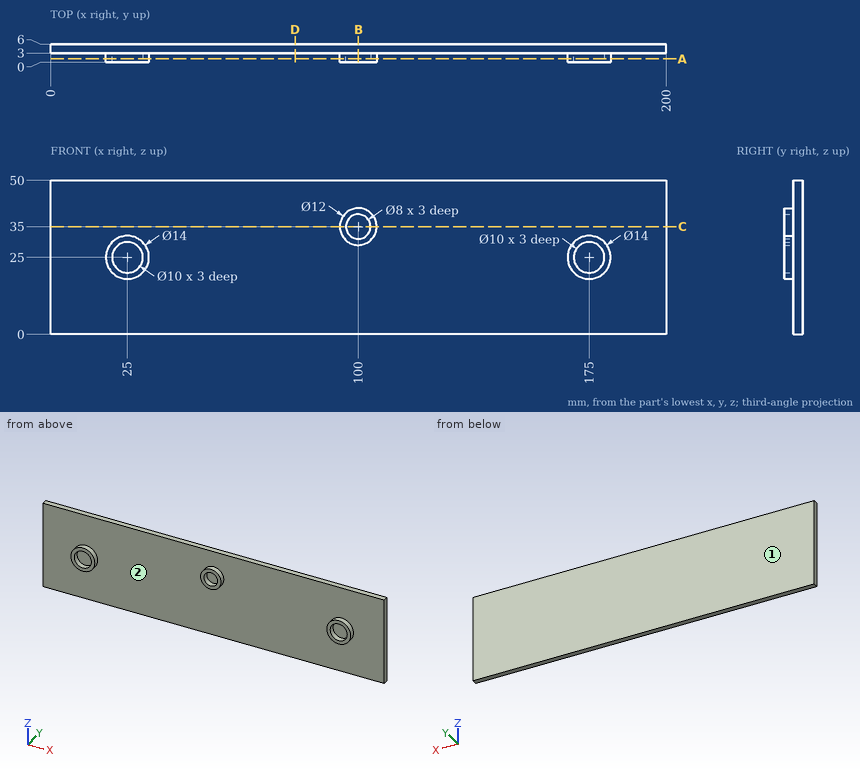
Could you check a few things on this drawing? It's one solid part, dimensions in mm from its lowest x, y, z. Round coordinates to 2 decimals unless told otherwise and drop trailing zeros. Order: outer loops, then holes, each group sorted by start corner. A loop starts at its lowest first (then second) coordinate and runs counter-clockwise, first axis right, second up. Notation, with made-up numbers: M 66,45 L 84,45 A12 cw 84,61 Z; hole C 85.5,41.5 d11. An arc over 180 degrees is marked long. One line per item, written item: value.
(1) I need wall thicknesses on line 1 along Z through (x, y) = (175, 2.2); line 2 along X through (y, z) = (1.35, 20.5); line 3 along Y through (x, z) = (16.5, 42.5). Which ranges of each line are inside material? Lowest first, please. Write a range as from..to.
Ans:
line 1: z = 18..20, 30..32
line 2: x = 19.64..22.82, 27.18..30.36, 169.64..172.82, 177.18..180.36
line 3: y = 3..6
(2) If we mould it in two halves opening along X, with no side actions, what happens to the marked faces 1 and 2? For each: released by +X, released by -X, zero draft, split by the parting line, or undercut.
Ans:
face 1: zero draft
face 2: undercut
(3) Imagine slicing it at C-C (z = 35). Write out the boundary of the cut face in (x, y).
Ans:
outline: M 0,3 L 94,3 L 94,0 L 96,0 L 96,3 L 104,3 L 104,0 L 106,0 L 106,3 L 200,3 L 200,6 L 0,6 Z
(4) Imagine slicing it at B-B (x = 100). Write out the boundary of the cut face in (y, z), and give its area (3 significant figures).
Ans:
outline: M 0,29 L 3,29 L 3,0 L 6,0 L 6,50 L 3,50 L 3,41 L 0,41 L 0,39 L 3,39 L 3,31 L 0,31 Z
area: 162 mm^2
(5) I'm going to push flat-ended pins straight in: P1, Ø2.5, axis at x = 101, z = 37, coming from the -Y side; P2, Ø5, axis at x = 22.5, z = 25.5, coming from the -Y side. Where does each tip first touch, or does it pass through?
Ans:
P1: stops at y = 3
P2: stops at y = 0
(6) Imagine slicing it at D-D (x = 79.5). Write out the boundary of the cut face in (y, z), and give its area (3 significant figures).
Ans:
outline: M 3,0 L 6,0 L 6,50 L 3,50 Z
area: 150 mm^2
(7) Imagine slicing it at A-A (y = 1.15). Write out the boundary of the cut face in (x, z).
Ans:
outline: C 25,25 d14; C 100,35 d12; C 175,25 d14; hole C 25,25 d10; hole C 100,35 d8; hole C 175,25 d10
